```python
from build123d import *

# Parameters (mm, degrees)
SALIENTE_EXTRUIR1_DEPTH      = 105
SALIENTE_EXTRUIR1_DEPTH_BACK = 0.1
CORTAR_EXTRUIR4_DEPTH        = 10
CROQUIS4_W                   = 0.15
CROQUIS4_H                   = 10
CORTAR_EXTRUIR9_DEPTH        = 0.1


with BuildPart() as part:
    # Croquis1 → Saliente-Extruir1 (new, two sides: drawn at the far end of the back side and taken through both)
    with BuildSketch(Plane(origin=(0, 0, 0), x_dir=(1, 0, 0), z_dir=(0, 1, 0)).offset(-SALIENTE_EXTRUIR1_DEPTH_BACK)):
        with BuildLine():
            Line((34.919955981, -1.488391566), (40.072080634, -1.226803632))
            add(Edge.make_bspline(
                [(40.072080634, -0.488391566), (40.190854748, -0.858541724), (40.072080634, -1.226803632)],
                knots=[0, 0, 0, 1, 1, 1], degree=2))
            Line((40.072080634, -0.488391566), (34.119955981, -0.488391566))
            ThreePointArc((34.119955981, -0.488391566), (33.766402591, -0.634838176), (33.619955981, -0.988391566))
            Line((33.619955981, -0.988391566), (33.619955981, -6.714416127))
            ThreePointArc((33.619955981, -6.714416127), (33.532088016, -6.926548161), (33.319955981, -7.014416127))
            Line((33.319955981, -7.014416127), (6.752124653, -7.014416127))
            ThreePointArc((6.752124653, -7.014416127), (6.539992619, -6.926548161), (6.452124653, -6.714416127))
            Line((6.452124653, -6.714416127), (6.452124653, -0.988391566))
            ThreePointArc((6.452124653, -0.988391566), (6.305678044, -0.634838176), (5.952124653, -0.488391566))
            Line((5.952124653, -0.488391566), (0, -0.488391566))
            add(Edge.make_bspline(
                [(0, -0.488391566), (-0.118774114, -0.858541724), (0, -1.226803632)],
                knots=[0, 0, 0, 1, 1, 1], degree=2))
            Line((0, -1.226803632), (5.152124653, -1.488391566))
            Line((5.152124653, -1.488391566), (5.152124653, -7.314416127))
            ThreePointArc((5.152124653, -7.314416127), (5.357149906, -7.809390874), (5.852124653, -8.014416127))
            Line((5.852124653, -8.014416127), (34.219955981, -8.014416127))
            ThreePointArc((34.219955981, -8.014416127), (34.714930728, -7.809390874), (34.919955981, -7.314416127))
            Line((34.919955981, -7.314416127), (34.919955981, -1.488391566))
        make_face()
    extrude(amount=SALIENTE_EXTRUIR1_DEPTH + SALIENTE_EXTRUIR1_DEPTH_BACK)

    # Croquis2 → Cortar-Extruir4 (cut)
    with BuildSketch(Plane.XY.offset(8.014416127)):
        with BuildLine():
            Line((16.786040317, 38.25), (16.786040317, 46.75))
            ThreePointArc((16.786040317, 46.75), (20.036040317, 50), (23.286040317, 46.75))
            Line((23.286040317, 46.75), (23.286040317, 38.25))
            ThreePointArc((23.286040317, 38.25), (20.036040317, 35), (16.786040317, 38.25))
        make_face()
        with BuildLine():
            Line((16.786040317, 13.25), (16.786040317, 21.75))
            ThreePointArc((16.786040317, 21.75), (20.036040317, 25), (23.286040317, 21.75))
            Line((23.286040317, 21.75), (23.286040317, 13.25))
            ThreePointArc((23.286040317, 13.25), (20.036040317, 10), (16.786040317, 13.25))
        make_face()
        with BuildLine():
            Line((16.786040317, 63.25), (16.786040317, 71.75))
            ThreePointArc((16.786040317, 71.75), (20.036040317, 75), (23.286040317, 71.75))
            Line((23.286040317, 71.75), (23.286040317, 63.25))
            ThreePointArc((23.286040317, 63.25), (20.036040317, 60), (16.786040317, 63.25))
        make_face()
        with BuildLine():
            Line((16.786040317, 88.25), (16.786040317, 96.75))
            ThreePointArc((16.786040317, 96.75), (20.036040317, 100), (23.286040317, 96.75))
            Line((23.286040317, 96.75), (23.286040317, 88.25))
            ThreePointArc((23.286040317, 88.25), (20.036040317, 85), (16.786040317, 88.25))
        make_face()
        with BuildLine():
            Line((16.786040317, 113.25), (16.786040317, 121.75))
            ThreePointArc((16.786040317, 121.75), (20.036040317, 125), (23.286040317, 121.75))
            Line((23.286040317, 121.75), (23.286040317, 113.25))
            ThreePointArc((23.286040317, 113.25), (20.036040317, 110), (16.786040317, 113.25))
        make_face()
        with BuildLine():
            Line((16.786040317, 138.25), (16.786040317, 146.75))
            ThreePointArc((16.786040317, 146.75), (20.036040317, 150), (23.286040317, 146.75))
            Line((23.286040317, 146.75), (23.286040317, 138.25))
            ThreePointArc((23.286040317, 138.25), (20.036040317, 135), (16.786040317, 138.25))
        make_face()
        with BuildLine():
            Line((16.786040317, 163.25), (16.786040317, 171.75))
            ThreePointArc((16.786040317, 171.75), (20.036040317, 175), (23.286040317, 171.75))
            Line((23.286040317, 171.75), (23.286040317, 163.25))
            ThreePointArc((23.286040317, 163.25), (20.036040317, 160), (16.786040317, 163.25))
        make_face()
        with BuildLine():
            Line((16.786040317, 188.25), (16.786040317, 196.75))
            ThreePointArc((16.786040317, 196.75), (20.036040317, 200), (23.286040317, 196.75))
            Line((23.286040317, 196.75), (23.286040317, 188.25))
            ThreePointArc((23.286040317, 188.25), (20.036040317, 185), (16.786040317, 188.25))
        make_face()
    extrude(amount=-CORTAR_EXTRUIR4_DEPTH, mode=Mode.SUBTRACT)

    # Croquis4 → Cortar-Extruir9 (cut)
    with BuildSketch(Plane(origin=(0, 0, 7.014416127), x_dir=(-1, 0, 0), z_dir=(0, 0, -1))):
        with Locations((-20.036040317, 29.95)):
            Rectangle(CROQUIS4_W, CROQUIS4_H)
        with Locations((-20.036040317, 4.95)):
            Rectangle(CROQUIS4_W, CROQUIS4_H)
        with Locations((-20.036040317, 54.95)):
            Rectangle(CROQUIS4_W, CROQUIS4_H)
        with Locations((-20.036040317, 79.95)):
            Rectangle(CROQUIS4_W, CROQUIS4_H)
        with Locations((-20.036040317, 104.95)):
            Rectangle(CROQUIS4_W, CROQUIS4_H)
        with Locations((-20.036040317, 129.95)):
            Rectangle(CROQUIS4_W, CROQUIS4_H)
        with Locations((-20.036040317, 154.95)):
            Rectangle(CROQUIS4_W, CROQUIS4_H)
        with Locations((-20.036040317, 179.95)):
            Rectangle(CROQUIS4_W, CROQUIS4_H)
    extrude(amount=-CORTAR_EXTRUIR9_DEPTH, mode=Mode.SUBTRACT)


solid = part.part
```
Part model, mm, in its own coordinate system. A direction names the side the tool comes from. Give positions to 0.01 mm unless a question says otherwise; leave off trailing zeros. Loops run counter-clockwise (first coordinate to the right, second up) from the corner with the lowest first, then second, coordinate; pieces in that order, holes last. Notation, with made-up numbers: M 31.25,89.5 L 61.25,89.5 A18 ccw 61.25,96.5 Z; hole C 28.25,33.25 d3. An arc over 180 degrees is marked long. Return JSON: item names as keys, results as strings.
1) Flat gauge pins, fed straight in: pin 1 Ø3 at (x, z) = (21.5, 5) entering from -Y; pin 2 Ø4 at (x, z) = (32.5, 2) entering from +Y; pin 3 Ø1.1 at (y, z) = (41.5, 7.5) entering from -X; pin 4 Ø3 at (y, z) = (35, 5.5) entering from +X. Where does each tip first touch, or does it go through?
Calculated:
{"pin 1": "passes through", "pin 2": "stops at y = 105", "pin 3": "stops at x = 5.15", "pin 4": "stops at x = 34.92"}
2) Saw through at A-A, the plane x = 12.5. List the corners of the cut face in (y, z), then the cut area to 3 significant figures.
Calculated:
{"outline": "M -0.1,7.01 L 105,7.01 L 105,8.01 L -0.1,8.01 Z", "area": "105 mm2"}
3) Drill centre lines: line 1 (X direction, y = 41.5, z = 5); line 2 (X direction, y = 89, z = 7.25); line 3 (Z direction, x = 14.5, y = 10). Where is each one in solid material? Low to high.
Calculated:
{"line 1": "x = 5.15 to 6.45, 33.62 to 34.92", "line 2": "x = 5.15 to 16.79, 23.29 to 34.92", "line 3": "z = 7.01 to 8.01"}
4) 3-axis set-ups, long thin cutter, end or side, ignore diameter. For faces 5 (the face through (5.152, 52, 4)), 6 (the face through (20.1, 60, 7.5)), 7 (the face through (23, 52, 7.014)), 8 (the face through (34.92, 52, 4)): which of +Z, -Z, +X, -X, +Y, -Y reach the whole face in a straight line?
Calculated:
{"face 5": "+Z, -X, +Y, -Y", "face 6": "+Z, -Z", "face 7": "-Z, +Y, -Y", "face 8": "+Z, +X, +Y, -Y"}
5) Pull direction Y, two halves, no side cores. Call faces 1 (the face through (33.62, 52, 4)), 2 (the face through (22.9, -0.1, 7.6)), 3 (the face through (20.1, 10, 7.5)), 4 (the face through (22.9, 105, 7.6)): released by +Y, released by -Y, zero draft, split by the parting line, or undercut.
Calculated:
{"face 1": "zero draft", "face 2": "released by -Y", "face 3": "undercut", "face 4": "released by +Y"}
6) Saw through at B-B, the plane x = 37.5. List the corners of the cut face in (y, z).
Calculated:
{"outline": "M -0.1,0.49 L 105,0.49 L 105,1.36 L -0.1,1.36 Z"}
